```python
from build123d import *

# Parameters (mm, degrees)
SKETCH1_W           = 50.8
SKETCH1_H           = 47
SKETCH1_R           = 0.75
BOSS_EXTRUDE1_DEPTH = 3
FILLET1_R           = 2.54


with BuildPart() as part:
    # Sketch1 → Boss-Extrude1 (new body)
    with BuildSketch(Plane(origin=(0, 0, 0), x_dir=(1, 0, 0), z_dir=(0, 1, 0))):
        Rectangle(SKETCH1_W, SKETCH1_H)
        with Locations((-22.86, 20.96)):
            Circle(SKETCH1_R, mode=Mode.SUBTRACT)
        with Locations((22.86, 20.96)):
            Circle(SKETCH1_R, mode=Mode.SUBTRACT)
        with Locations((22.86, -20.96)):
            Circle(SKETCH1_R, mode=Mode.SUBTRACT)
        with Locations((-22.86, -20.96)):
            Circle(SKETCH1_R, mode=Mode.SUBTRACT)
        with Locations((10, 0)):
            Circle(SKETCH1_R, mode=Mode.SUBTRACT)
        with Locations((-10, 0)):
            Circle(SKETCH1_R, mode=Mode.SUBTRACT)
    extrude(amount=BOSS_EXTRUDE1_DEPTH)

    # Fillet1
    fillet1_edges = [part.edges().sort_by_distance(p)[0] for p in [
        (-25.4, 1.5, -23.5),
        (25.4, 1.5, -23.5),
        (25.4, 1.5, 23.5),
        (-25.4, 1.5, 23.5),
    ]]
    fillet(fillet1_edges, radius=FILLET1_R)


solid = part.part
```
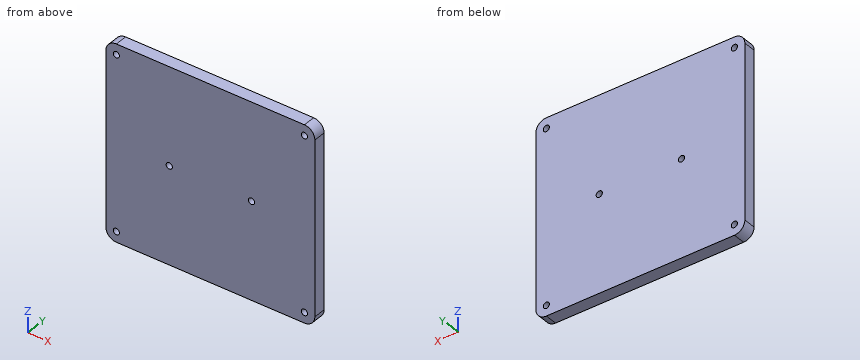
For this review, take the finished solid that the model builds, in its own axes (mm). Round coordinates to 2 decimals unless told otherwise and drop trailing zeros. Order: outer loops, then holes, each group sorted by start corner. A loop starts at its lowest first (then second) coordinate and runs counter-clockwise, first axis right, second up. Notation, with made-up numbers: (-19, 12) -> (9, 12) arc R31 cw to (9, 39) -> close; hole circle Ø8 at (30.5, -3). An arc over 180 degrees is marked (long way). Use a Markdown table: item, result.
Item 1: For pin 1 (0.9 mm diameter, centred on x = 10, z = 0, fed in from -Y), flat-tipped, find the tip position at first contact; note if it passes through.
Resolved:
| item | result |
|---|---|
| pin 1 | passes through |
Item 2: Take a section at B-B (z = 0). State the section outline as (x, y) points, plus the area to 3 significant figures.
Resolved:
| item | result |
|---|---|
| outline | (-25.4, 0) -> (-10.75, 0) -> (-10.75, 3) -> (-25.4, 3) -> close; (-9.25, 0) -> (9.25, 0) -> (9.25, 3) -> (-9.25, 3) -> close; (10.75, 0) -> (25.4, 0) -> (25.4, 3) -> (10.75, 3) -> close |
| area | 143 mm² |
Item 3: Take a section at A-A (x = 10). State the section outline as (y, z) points.
Resolved:
| item | result |
|---|---|
| outline | (0, -23.5) -> (3, -23.5) -> (3, -0.75) -> (0, -0.75) -> close; (0, 0.75) -> (3, 0.75) -> (3, 23.5) -> (0, 23.5) -> close |
Item 4: For line 1 along Z through (x, y) = (22.86, 2.05); line 2 along X through (y, z) = (2.2, 0); line 3 along X through (y, z) = (2.2, 20.96), list the stretches that pass through material, from the lowest coordinate up. Write a range as [from, to].
Resolved:
| item | result |
|---|---|
| line 1 | z = [-23.5, -21.71], [-20.21, 20.21], [21.71, 23.5] |
| line 2 | x = [-25.4, -10.75], [-9.25, 9.25], [10.75, 25.4] |
| line 3 | x = [-25.4, -23.61], [-22.11, 22.11], [23.61, 25.4] |
